Verification items for the finished model (mm, model axes). A direction names the side the tool comes from. Coordinates: 2 decimals unless noted, no trailing zeros. Write each loop counter-clockwise with the first axis right and the second up, starting at its lowest first coordinate (ties: lowest second). Pieces come first, ordered by that corner, then holes. Notation, with made-up numbers: (48, 57.25) -> (62, 57.25) arc R23 ccw to (62, 89.25) -> close; hole circle Ø11 at (65.5, 39). An arc over 180 degrees is marked (long way). Answer in a Markdown table with one row per item.
```python
from build123d import *

# Parameters (mm, degrees)
CROQUIS2_R              = 3.1
SALIENTE_EXTRUIR1_DEPTH = 3
CROQUIS4_R              = 2.1
SALIENTE_EXTRUIR2_DEPTH = 6
REDONDEO1_R             = 5


with BuildPart() as part:
    # Croquis2 → Saliente-Extruir1 (new, symmetric)
    with BuildSketch(Plane(origin=(0, 58.707138557, 0), x_dir=(1, 0, 0), z_dir=(0, 1, 0))):
        Polygon((-236.097571291, -325), (-242.097571291, -325), (-242.097571291, -205), (-236.097571291, -205), (-216.097571291, -205), (-216.097571291, -225), (-236.097571291, -225), (-236.097571291, -255), (-216.097571291, -255), (-216.097571291, -275), (-236.097571291, -275), (-236.097571291, -305), (-216.097571291, -305), (-216.097571291, -325), align=None)
        with Locations(Location((-224.097571291, -215, 0), (0, 0, 270))):
            Circle(CROQUIS2_R, mode=Mode.SUBTRACT)
        with Locations(Location((-224.097571291, -265, 0), (0, 0, 270))):
            Circle(CROQUIS2_R, mode=Mode.SUBTRACT)
        with Locations(Location((-224.097571291, -315, 0), (0, 0, 270))):
            Circle(CROQUIS2_R, mode=Mode.SUBTRACT)
    extrude(amount=SALIENTE_EXTRUIR1_DEPTH, both=True)

    # Croquis4 → Saliente-Extruir2 (add)
    with BuildSketch(Plane.ZY.offset(242.097571291)):
        Polygon((205, 61.707138557), (325, 61.707138557), (305, 101.707138557), (225, 101.707138557), align=None)
        with Locations((250.49, 66.952138557)):
            Circle(CROQUIS4_R, mode=Mode.SUBTRACT)
        with Locations((229.49, 66.952138557)):
            Circle(CROQUIS4_R, mode=Mode.SUBTRACT)
        with Locations((279.49, 66.952138557)):
            Circle(CROQUIS4_R, mode=Mode.SUBTRACT)
        with Locations((300.49, 66.952138557)):
            Circle(CROQUIS4_R, mode=Mode.SUBTRACT)
        with Locations((279.49, 94.952138557)):
            Circle(CROQUIS4_R, mode=Mode.SUBTRACT)
        with Locations((300.49, 94.952138557)):
            Circle(CROQUIS4_R, mode=Mode.SUBTRACT)
        with Locations((229.49, 94.952138557)):
            Circle(CROQUIS4_R, mode=Mode.SUBTRACT)
        with Locations((250.49, 94.952138557)):
            Circle(CROQUIS4_R, mode=Mode.SUBTRACT)
    extrude(amount=-SALIENTE_EXTRUIR2_DEPTH)

    # Redondeo1
    redondeo1_edges = [part.edges().sort_by_distance(p)[0] for p in [
        (-242.097571291, 55.707138557, 265),
        (-216.097571291, 58.707138557, 205),
        (-216.097571291, 58.707138557, 225),
        (-216.097571291, 58.707138557, 255),
        (-216.097571291, 58.707138557, 275),
        (-216.097571291, 58.707138557, 305),
        (-216.097571291, 58.707138557, 325),
        (-239.097571291, 101.707138557, 305),
        (-239.097571291, 101.707138557, 225),
    ]]
    fillet(redondeo1_edges, radius=REDONDEO1_R)


solid = part.part
```
1. Access from +Z, -Z, +X, -X, +Y, -Y to the whole of each face (thin tool, end or side, straight path). Record for faces 4 (the face through (-228, 61.707, 265)), 5 (the face through (-228, 59, 225)), 6 (the face through (-217.601, 58.749, 323.574)).
Findings below:
| item | result |
|---|---|
| face 4 | +Z, -Z, +X, +Y |
| face 5 | +X, +Y, -Y |
| face 6 | +Z, +X, +Y, -Y |
2. Release check for a two-part mould opening along Y. For faces 1 (the face through (-216.098, 59, 265)), 2 (the face through (-239.14, 66.15, 252.43)), 3 (the face through (-229, 55.707, 264)) record: released by +Y, released by -Y, zero draft, split by the parting line, or undercut.
Findings below:
| item | result |
|---|---|
| face 1 | zero draft |
| face 2 | undercut |
| face 3 | released by -Y |
3. Sectioned sample at A-A, the plane z = 265. Record the cut outline in (x, y).
Findings below:
| item | result |
|---|---|
| outline | (-242.1, 60.71) arc R5 ccw to (-237.1, 55.71) -> (-227.2, 55.71) -> (-227.2, 61.71) -> (-236.1, 61.71) -> (-236.1, 101.71) -> (-242.1, 101.71) -> close; (-221, 55.71) -> (-216.1, 55.71) -> (-216.1, 61.71) -> (-221, 61.71) -> close |
4. Sectioned sample at D-D, the plane z = 315. Record the cut outline in (x, y), and give its area (3 significant figures).
Findings below:
| item | result |
|---|---|
| outline | (-242.1, 60.71) arc R5 ccw to (-237.1, 55.71) -> (-227.2, 55.71) -> (-227.2, 61.71) -> (-236.1, 61.71) -> (-236.1, 81.71) -> (-242.1, 81.71) -> close; (-221, 55.71) -> (-216.1, 55.71) -> (-216.1, 61.71) -> (-221, 61.71) -> close |
| area | 233 mm² |
5. Sectioned sample at B-B, the plane z = 229.49. Record the cut outline in (x, y).
Findings below:
| item | result |
|---|---|
| outline | (-242.1, 60.71) arc R5 ccw to (-237.1, 55.71) -> (-236.1, 55.71) -> (-236.1, 64.85) -> (-242.1, 64.85) -> close; (-242.1, 69.05) -> (-236.1, 69.05) -> (-236.1, 92.85) -> (-242.1, 92.85) -> close; (-242.1, 97.05) -> (-236.1, 97.05) -> (-236.1, 101.71) -> (-242.1, 101.71) -> close |
6. Sectioned sample at C-C, the plane z = 294. Record the cut outline in (x, y), and give its area (3 significant figures).
Findings below:
| item | result |
|---|---|
| outline | (-242.1, 60.71) arc R5 ccw to (-237.1, 55.71) -> (-236.1, 55.71) -> (-236.1, 101.71) -> (-242.1, 101.71) -> close |
| area | 271 mm² |
7. Go/stop test with flat-tipped pins: pin 1 (3.5 mm diameter, centred on x = -224.1, z = 315, fed in from -Y); pin 2 (6.5 mm diameter, centred on y = 66.95, z = 250.49, fed in from +X); pin 3 (6 mm diameter, centred on x = -227.5, z = 264.5, fed in from +Y); pin 4 (1.5 mm diameter, centred on x = -239.5, y = 82, fed in from +Z). Record where each tip stops, or that it passes through.
Findings below:
| item | result |
|---|---|
| pin 1 | passes through |
| pin 2 | stops at x = -236.1 |
| pin 3 | stops at y = 61.71 |
| pin 4 | stops at z = 315.23 |
8. Material ranges on probe 1 along Y at (x, z) = (-238.55, 300.49); probe 2 along Y at (x, z) = (-237.6, 279.49); probe 3 along X at (y, z) = (68, 264), recorded low to high. Write a range as from..to.
Findings below:
| item | result |
|---|---|
| probe 1 | y = 55.92..64.85, 69.05..92.85, 97.05..101.71 |
| probe 2 | y = 55.73..64.85, 69.05..92.85, 97.05..101.71 |
| probe 3 | x = -242.1..-236.1 |
